from build123d import *

# Parameters (mm, degrees)
LPATTERN1_COUNT                     = 2
LPATTERN1_PITCH                     = 12.7
F_3_16_0_1875_DIAMETER_HOLE1_REACH  = 102.34
F_3_16_0_1875_DIAMETER_HOLE1_BORE_R = 2.38125
CIRPATTERN1_COUNT                   = 8


with BuildPart() as part:
    # Sketch1 → Revolve1 (revolve)
    with BuildSketch(Plane.XY, mode=Mode.PRIVATE) as revolve1_sk:
        Polygon((-41.275, 13.97), (-41.275, 45.72), (-34.925, 45.72), (-34.925, 26.67), (-2.2098, 26.67), (-2.2098, 1.4986), (-3.683, 0.0254), (-3.683, 0), (-5.1435, 0), (-5.1435, 13.97), (-34.925, 13.97), (-34.925, 0), (-41.275, 0), align=None)
    revolve(revolve1_sk.sketch.rotate(Axis((0, 0, 0), (0, 1, 0)), 270), axis=Axis((0, 0, 0), (0, 1, 0)))

    # Sketch3 → Groove for AS 568-234, O-Ring1 (revolve, cut)
    with BuildSketch(Plane(origin=(0, 0, 0), x_dir=(0, 0, -1), z_dir=(-1, 0, 0)), mode=Mode.PRIVATE) as groove_for_as_568_234_o_ring1_sk:
        with BuildLine():
            Line((38.861359272, -30.6451), (41.3639, -30.426156056))
            Line((41.3639, -30.426156056), (41.3639, -35.613843944))
            Line((41.3639, -35.613843944), (38.861359272, -35.3949))
            ThreePointArc((38.861359272, -35.3949), (38.572380224, -35.252391304), (38.4556, -34.952091457))
            Line((38.4556, -34.952091457), (38.4556, -31.087908543))
            ThreePointArc((38.4556, -31.087908543), (38.572380224, -30.787608696), (38.861359272, -30.6451))
        make_face()
    groove_for_as_568_234_o_ring1 = revolve(groove_for_as_568_234_o_ring1_sk.sketch.rotate(Axis((0, -50, 0), (0, 1, 0)), 180), axis=Axis((0, -50, 0), (0, 1, 0)), mode=Mode.SUBTRACT)

    # LPattern1: Groove for AS 568-234, O-Ring1 ×2
    with Locations(*[(0, -i * LPATTERN1_PITCH, 0) for i in range(1, LPATTERN1_COUNT)]):
        add(groove_for_as_568_234_o_ring1, mode=Mode.SUBTRACT)

    # 3/16 (0.1875) Diameter Hole1 bore (on position points) → 3/16 (0.1875) Diameter Hole1 (cut, up to next)
    with BuildSketch(Plane(origin=(41.275, 6.35, 0), x_dir=(0, 0, 1), z_dir=(1, 0, 0)), mode=Mode.PRIVATE) as f_3_16_0_1875_diameter_hole1_sk1:
        Circle(F_3_16_0_1875_DIAMETER_HOLE1_BORE_R)
    f_3_16_0_1875_diameter_hole1_tool1 = extrude(f_3_16_0_1875_diameter_hole1_sk1.sketch, amount=-F_3_16_0_1875_DIAMETER_HOLE1_REACH, mode=Mode.PRIVATE) & part.part
    f_3_16_0_1875_diameter_hole1 = f_3_16_0_1875_diameter_hole1_tool1.solids().sort_by_distance((41.275, 6.35, 0))[0]
    add(f_3_16_0_1875_diameter_hole1, mode=Mode.SUBTRACT)

    # CirPattern1: 3/16 (0.1875) Diameter Hole1 ×8 about axis
    cirpattern1_axis = Axis((0, -2.286, 0), (0, 1, 0))
    for i in range(1, CIRPATTERN1_COUNT):
        add(f_3_16_0_1875_diameter_hole1.rotate(cirpattern1_axis, i * 360 / CIRPATTERN1_COUNT), mode=Mode.SUBTRACT)


solid = part.part
Here's how the part is built. I have some questions about the finished solid (model axes, mm). A direction names the side the tool comes from. Coordinates: 2 decimals unless noted, no trailing zeros.
1. If we mould it in two halves opening along X, with no side actions, what happens to faces 1 (the cylindrical face through (-37.54, 20.29, -8.34)), 2 (the flat face through (-9, 0, -34)), 3 (the cylindrical face through (34.094, 36.062, 7.571))? For each: pulls with the +X half, pulls with the -X half, needs draft (parallel to the pull), parting line crosses it, or undercut.
2. For P1, Ø12, axis at x = 1, z = 1.5, coming from the +Y side; P2, Ø2, axis at x = 31.5, y = 12.5, coming from the -Z side; P3, Ø3, axis at x = 0, y = 6.35, coming from the +Z side, each with a flat end and sliding along its axis, tell me the tip position at first contact or that it passes through.
3. I need wall thicknesses on L1, parallel to X at y = 0.05, z = 0 (1 decimal); L2, parallel to X at y = 9.5, z = 0 (1 decimal); L3, parallel to X at y = 40, z = 0 (3 decimals). Which ranges of each line are inside material? Lowest first, please.
4. Imagine slicing it at A-A, the plane y = 6.35. Count the separate pieces of the cut face and the enclosed holes in it, and give its area (3 significant figures).
5. For faces 4 (the conical face through (11.72, 17.93, 37.21)), 5 (the cylindrical face through (-38.1, 3.99, 0.31)), 6 (the cylindrical face through (-0.31, 3.99, -38.1)), 7 (the cylindrical face through (13.38, 6.89, -32.26)), which set-ups out of +Z, -Z, +X, -X, +Y, -Y let a thin tool reach every point of the face, with its end or its side?
Taken from the geometry:
1. face 1: parting line crosses it
1. face 2: needs draft
1. face 3: undercut
2. P1: stops at y = 26.67
2. P2: stops at z = -27.81
2. P3: stops at z = 5.14
3. L1: x = -41.3 to -34.9, -5.1 to -3.7, 3.7 to 5.1, 34.9 to 41.3
3. L2: x = -41.3 to -34.9, -5.1 to -2.2, 2.2 to 5.1, 34.9 to 41.3
3. L3: x = -41.275 to -34.925, 34.925 to 41.275
4. separate pieces: 9
4. enclosed holes: 1
4. area: 1,350 mm2
5. face 4: none
5. face 5: -X
5. face 6: -Z
5. face 7: -Y
